```python
from build123d import *

# Parameters (mm, degrees)
F0_W     = 59
F0_H     = 59
F1_DEPTH = 55
F2_R     = 10
F3_T     = -2
F5_DEPTH = 25
F6_R     = 1.75
F7_DEPTH = 20
F8_R     = 2


with BuildPart() as f1:
    # F0 (on Front) → F1 (new body)
    with BuildSketch(Plane.XZ):
        Rectangle(F0_W, F0_H)
    extrude(amount=F1_DEPTH)

    # F2
    f2_edges = [f1.edges().sort_by_distance(p)[0] for p in [
        (-29.5, -27.5, 29.5),
        (29.5, -27.5, 29.5),
        (29.5, -27.5, -29.5),
        (-29.5, -27.5, -29.5),
        (29.5, 0, 0),
        (0, 0, 29.5),
        (0, 0, -29.5),
        (-29.5, 0, 0),
    ]]
    fillet(f2_edges, radius=F2_R)

    # F3
    f3_openings = [f1.faces().sort_by_distance(p)[0] for p in [
        (0, -55, 0),
    ]]
    offset(amount=F3_T, openings=f3_openings)

    # F4 (on face) → F5 (join)
    with BuildSketch(Plane.XZ.offset(55)):
        with BuildLine():
            ThreePointArc((-29.5, 19.5), (-26.571068, 26.571068), (-19.5, 29.5))
            Line((-19.5, 29.5), (-29.5, 29.5))
            Line((-29.5, 29.5), (-29.5, 19.5))
        make_face()
        with BuildLine():
            Line((29.5, 29.5), (19.5, 29.5))
            ThreePointArc((19.5, 29.5), (26.571068, 26.571068), (29.5, 19.5))
            Line((29.5, 19.5), (29.5, 29.5))
        make_face()
        with BuildLine():
            Line((-29.5, -19.5), (-29.5, -29.5))
            Line((-29.5, -29.5), (-19.5, -29.5))
            ThreePointArc((-19.5, -29.5), (-26.571068, -26.571068), (-29.5, -19.5))
        make_face()
        with BuildLine():
            ThreePointArc((29.5, -19.5), (26.571068, -26.571068), (19.5, -29.5))
            Line((19.5, -29.5), (29.5, -29.5))
            Line((29.5, -29.5), (29.5, -19.5))
        make_face()
        with BuildLine():
            Line((-27.5, -2.5), (-26.25, -2.5))
            ThreePointArc((-26.25, -2.5), (-23.75, 0), (-26.25, 2.5))
            Line((-26.25, 2.5), (-27.5, 2.5))
            Line((-27.5, 2.5), (-27.5, -2.5))
        make_face()
        with BuildLine():
            ThreePointArc((26.25, 2.5), (23.75, 0), (26.25, -2.5))
            Line((26.25, -2.5), (27.5, -2.5))
            Line((27.5, -2.5), (27.5, 2.5))
            Line((27.5, 2.5), (26.25, 2.5))
        make_face()
    extrude(amount=-F5_DEPTH)

    # F6 (on face) → F7 (cut)
    with BuildSketch(Plane.XZ.offset(55)):
        with Locations((27.136753, 27.136753)):
            Circle(F6_R)
        with Locations((27.136753, -27.136753)):
            Circle(F6_R)
        with Locations((-27.136753, -27.136753)):
            Circle(F6_R)
        with Locations((-27.136753, 27.136753)):
            Circle(F6_R)
        with Locations((-26.25, 0)):
            Circle(F6_R)
        with Locations((26.25, 0)):
            Circle(F6_R)
    extrude(amount=-F7_DEPTH, mode=Mode.SUBTRACT)

    # F8
    f8_edges = [f1.edges().sort_by_distance(p)[0] for p in [
        (29.5, -42.5, 29.5),
        (29.5, -42.5, -29.5),
        (-29.5, -42.5, 29.5),
        (-29.5, -42.5, -29.5),
    ]]
    fillet(f8_edges, radius=F8_R)


solid = f1.part
```
CAD build for the part. Positions are in the model's coordinates, mm. A direction names the side the tool comes from. Give positions to 0.01 mm unless a question says otherwise; leave off trailing zeros. Order: outer loops, then holes, each group sorted by start corner. A loop starts at its lowest first (then second) coordinate and runs counter-clockwise, first axis right, second up. Notation, with made-up numbers: M 23,3.5 L 72,3.5 A19 ccw 72,18.5 Z; hole C -3.75,3 d11. An arc over 180 degrees is marked long. Put each result on its own line as item: value. Start each with the question number.
(1) Drill centre lines: line 1 along X through (y, z) = (-34.5, 7); line 2 along Y through (x, z) = (-2, -2.5). Where is each one in solid material? Low to high.
(2) Flat gauge pins, fed straight in: pin 1 Ø11.5 at (x, z) = (2.5, 0.5) entering from -Y; pin 2 Ø12 at (x, y) = (-1.5, -8.5) entering from +Z; pin 3 Ø3 at (x, z) = (27.14, -27.14) entering from -Y; pin 4 Ø5 at (x, z) = (-24, 24.5) entering from +Y. Where does each tip first touch, or does it go through?
(3) Saw through at C-C, the plane y = -52. Give the number of separate pieces and of enclosed holes in the cut face, then the cut area to 3 significant figures.
(4) Mould opens along X. For faces 1 (the flat face through (-26, -35, 0)), 2 (the flat face through (-27, -35, -27)), 3 (the cylindrical face through (28.93, -42.32, -28.9)), 4 (the cylindrical face through (-28.93, -42.32, -28.9)) say: +X half, -X half, draft (parallel to the pull), parting line (faces both ways), or undercut.
(5) Saw through at B-B, the plane z = 0. Write the cut outline in (x, y), then the cut area to 3 significant figures.
(6) Saw through at A-A, the plane y = -25. Write the cut outline in (x, z), then the cut area to 3 significant figures.
(7) Which spindle directions (+Z, -Z, +X, -X, +Y, -Y) get a long thin tool onto all of the face, cutting with end or side? Do faces 5 (the cylindrical face through (-26.65, -20.14, -26.49)), 6 (the flat face through (27, -30, 27)), 7 (the cylindrical face through (0.273, -4.406, 25.219)). Say none if no direction does.
(8) Saw through at D-D, the plane x = -10. Write the cut outline in (y, z).
Check result:
1. line 1: x = -29.5 to -27.5, 27.5 to 29.5
1. line 2: y = -2 to 0
2. pin 1: stops at y = -2
2. pin 2: stops at z = 29.5
2. pin 3: stops at y = -35
2. pin 4: stops at y = -0.94
3. separate pieces: 1
3. enclosed holes: 7
3. area: 482 mm2
4. face 1: undercut
4. face 2: undercut
4. face 3: +X half
4. face 4: -X half
5. outline: M -29.5,-55 L -28,-55 L -28,-35 L -24.5,-35 L -24.5,-55 L -23.75,-55 L -23.75,-30 L -27.5,-30 L -27.5,-10 A8 cw -19.5,-2 L 19.5,-2 A8 cw 27.5,-10 L 27.5,-30 L 23.75,-30 L 23.75,-55 L 24.5,-55 L 24.5,-35 L 28,-35 L 28,-55 L 29.5,-55 L 29.5,-10 A10 ccw 19.5,0 L -19.5,0 A10 ccw -29.5,-10 Z
5. area: 362 mm2
6. outline: M -29.5,-19.5 A10 ccw -19.5,-29.5 L 19.5,-29.5 A10 ccw 29.5,-19.5 L 29.5,19.5 A10 ccw 19.5,29.5 L -19.5,29.5 A10 ccw -29.5,19.5 Z; hole M -27.5,-19.5 A8 ccw -19.5,-27.5 L 19.5,-27.5 A8 ccw 27.5,-19.5 L 27.5,19.5 A8 ccw 19.5,27.5 L -19.5,27.5 A8 ccw -27.5,19.5 Z
6. area: 425 mm2
7. face 5: -Z, -X, +Y
7. face 6: +Z, +X, +Y
7. face 7: -Y
8. outline: M -55,-29.5 L -10,-29.5 A10 ccw 0,-19.5 L 0,19.5 A10 ccw -10,29.5 L -55,29.5 L -55,27.5 L -10,27.5 A8 cw -2,19.5 L -2,-19.5 A8 cw -10,-27.5 L -55,-27.5 Z
